For this review, take the finished solid that the model builds, in its own axes (mm). Face numbers are marked on the shaded views. A direction names the side the tool comes from. Give positions to 0.01 mm unless a question says otherwise; leave off trailing zeros. Order: outer loops, then holes, each group sorted by start corner. A loop starts at its lowest first (then second) coordinate and runs counter-clockwise, first axis right, second up. Notation, with made-up numbers: (-34, 76.25) - (-4, 76.25) arc R20 ccw to (-4, 103.25) - close; hole circle Ø6 at (-24.75, 33). An arc over 180 degrees is marked (long way). One line per item, written item: value.
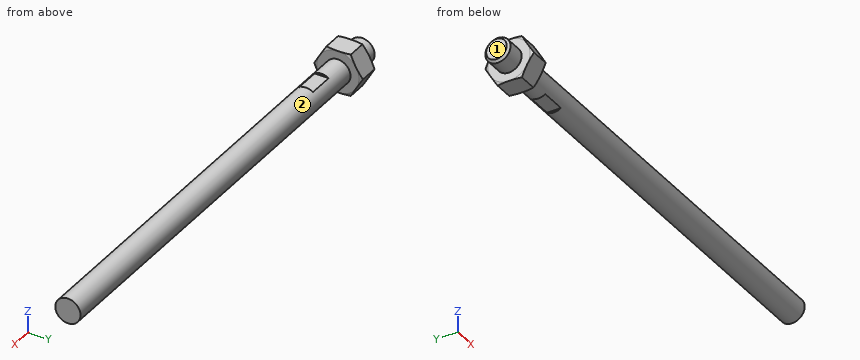
```python
from build123d import *

# Parameters (mm, degrees)
EXTRUDE_START        = -38
SKETCH_3_R           = 3
EXTRUDE_1_DEPTH      = 16
EXTRUDE_START_2      = -33.2
EXTRUDE_2_DEPTH      = 5
SKETCH_5_R           = 3
EXTRUDE_3_DEPTH      = 97
CUT_EXTRUDE_START    = -22
SKETCH_6_OUTSIDE_W   = 34.806
SKETCH_6_OUTSIDE_H   = 36.354
SKETCH_6_OUTSIDE_W_2 = 5
SKETCH_6_OUTSIDE_H_2 = 11.547005384
CUT_EXTRUDE_1_DEPTH  = 6
CHAMFER_1_SIZE       = 0.56


with BuildPart() as part:
    # 草图3 → 凸台-拉伸1 (new body)
    with BuildSketch(Plane(origin=(0, 0, 0), x_dir=(0, 0, -1), z_dir=(1, 0, 0)).offset(EXTRUDE_START)):
        Circle(SKETCH_3_R)
    extrude(amount=EXTRUDE_1_DEPTH)

    # 草图4 → 凸台-拉伸2 (add)
    with BuildSketch(Plane(origin=(0, 0, 0), x_dir=(0, 0, -1), z_dir=(1, 0, 0)).offset(EXTRUDE_START_2)):
        Polygon((0, -5.773502692), (5, -2.886751346), (5, 2.886751346), (0, 5.773502692), (-5, 2.886751346), (-5, -2.886751346), align=None)
    extrude(amount=EXTRUDE_2_DEPTH)

    # 草图5 → 凸台-拉伸3 (add)
    with BuildSketch(Plane(origin=(-22, 0, 0), x_dir=(0, 0, -1), z_dir=(1, 0, 0))):
        Circle(SKETCH_5_R)
    extrude(amount=EXTRUDE_3_DEPTH)

    # 草图6 outside → 切除-拉伸1 (cut)
    with BuildSketch(Plane(origin=(0, 0, 0), x_dir=(0, 0, -1), z_dir=(1, 0, 0)).offset(CUT_EXTRUDE_START)):
        Rectangle(SKETCH_6_OUTSIDE_W, SKETCH_6_OUTSIDE_H)
        Rectangle(SKETCH_6_OUTSIDE_W_2, SKETCH_6_OUTSIDE_H_2, mode=Mode.SUBTRACT)
    extrude(amount=CUT_EXTRUDE_1_DEPTH, mode=Mode.SUBTRACT)

    # 草图7 → 切除-旋转1 (revolve, cut)
    with BuildSketch(Plane(origin=(0, 0, 0), x_dir=(1, 0, 0), z_dir=(0, 1, 0))):
        Polygon((-33.2, 5), (-33.2, 16.868693549), (-28.2, 16.868693549), (-28.2, 5), (-30.7, 11.868693549), align=None)
    revolve(axis=Axis((-16, 0, 0), (-1, 0, 0)), mode=Mode.SUBTRACT)

    # 倒角1
    chamfer_1_edges = [part.edges().sort_by_distance(p)[0] for p in [
        (-38, 0, 3),
    ]]
    chamfer(chamfer_1_edges, length=CHAMFER_1_SIZE)


solid = part.part
```
(1) Wall thickness on line 1 (Y direction, x = 32.5, z = 0.25); line 2 (X direction, y = 4, z = 2.75); line 3 (Y direction, x = 29, z = -1.75): over which ranges is each line inside the solid? List them lowest first. Write a range as from..to.
Answers below:
line 1: y = -2.99..2.99
line 2: x = -33.2..-28.2
line 3: y = -2.44..2.44
(2) Take a section at A-A (x = 32). Write out the cut boundary in (y, z), then the cut area to 3 significant figures.
Answers below:
outline: circle Ø6 at (0, 0)
area: 28.3 mm^2
(3) Machinability: for the marked faces 1 and 2, which of the approach directions +Z, -Z, +X, -X, +Y, -Y give a long, thin tool a straight path to every point of the face, cutting with its end or side? Answer none if there is none.
Answers below:
face 1: +Z, -Z, -X, +Y, -Y
face 2: +X
(4) For P1, Ø2, axis at x = 61.5, z = -3.5, coming from the +Y side; P2, Ø5, axis at x = 16, y = -2.5, coming from the +Z side; P3, Ø3, axis at x = 52.5, y = -3, coming from the +Z side, all flat-tipped, find the tip position at first contact; note any pin that passes through.
Answers below:
P1: stops at y = 1.66
P2: stops at z = 3
P3: stops at z = 2.6
